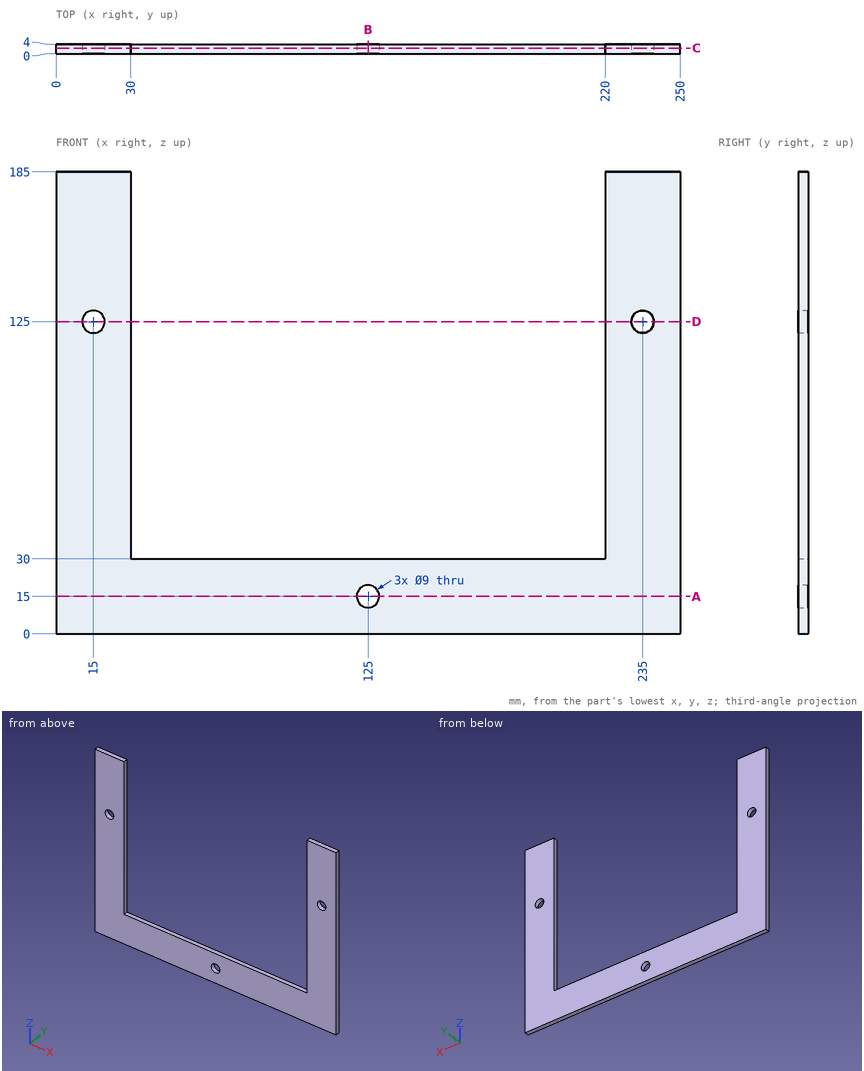
For this review, use the dimensioned drawing (mm, ordinates from the lowest corner) and the shaded views. Coordinates: 2 decimals unless noted, no trailing zeros. Order: outer loops, then holes, each group sorted by start corner. A loop starts at its lowest first (then second) coordinate and runs counter-clockwise, first axis right, second up. Notation, with made-up numbers: (2, 31.5) -> (23, 31.5) arc R21 ccw to (23, 62.5) -> close; hole circle Ø9 at (13.5, 0). An arc over 180 degrees is marked (long way). One line per item, written item: value. Start each with the question number.
Q1. Take a section at A-A, the plane z = 15. State the section outline as (x, y) points, then the cut area to 3 significant figures.
Q2. Take a section at D-D, the plane z = 125. State the section outline as (x, y) points, then the cut area to 3 significant figures.
Q3. Take a section at B-B, the plane x = 125. State the section outline as (y, z) points, then the cut area to 3 significant figures.
Q4. Take a section at C-C, the plane y = 2.3. State the section outline as (x, z) points.
Q5. Insertion check: pin 1 Ø8 at (x, z) = (235, 125) entering from -Y; pin 2 Ø1 at (x, y) = (132.5, 3.5) entering from +Z. Each pin has a flat end and moves straight along its axis. Give the tip position at first contact, or say it passes through.
Q6. For probe 1 along X at (y, z) = (2, 125); probe 2 along X at (y, z) = (1.65, 73); probe 3 along X at (y, z) = (3.05, 122), list the stretches that pass through material, from the lowest coordinate up.
Values follow:
1. outline: (0, 0) -> (120.5, 0) -> (120.5, 4) -> (0, 4) -> close; (129.5, 0) -> (250, 0) -> (250, 4) -> (129.5, 4) -> close
1. area: 964 mm2
2. outline: (0, 0) -> (10.5, 0) -> (10.5, 4) -> (0, 4) -> close; (19.5, 0) -> (30, 0) -> (30, 4) -> (19.5, 4) -> close; (220, 0) -> (230.5, 0) -> (230.5, 4) -> (220, 4) -> close; (239.5, 0) -> (250, 0) -> (250, 4) -> (239.5, 4) -> close
2. area: 168 mm2
3. outline: (0, 0) -> (4, 0) -> (4, 10.5) -> (0, 10.5) -> close; (0, 19.5) -> (4, 19.5) -> (4, 30) -> (0, 30) -> close
3. area: 84.0 mm2
4. outline: (0, 0) -> (250, 0) -> (250, 185) -> (220, 185) -> (220, 30) -> (30, 30) -> (30, 185) -> (0, 185) -> close; hole circle Ø9 at (15, 125); hole circle Ø9 at (125, 15); hole circle Ø9 at (235, 125)
5. pin 1: passes through
5. pin 2: stops at z = 30
6. probe 1: x = 0 to 10.5, 19.5 to 30, 220 to 230.5, 239.5 to 250
6. probe 2: x = 0 to 30, 220 to 250
6. probe 3: x = 0 to 11.65, 18.35 to 30, 220 to 231.65, 238.35 to 250
